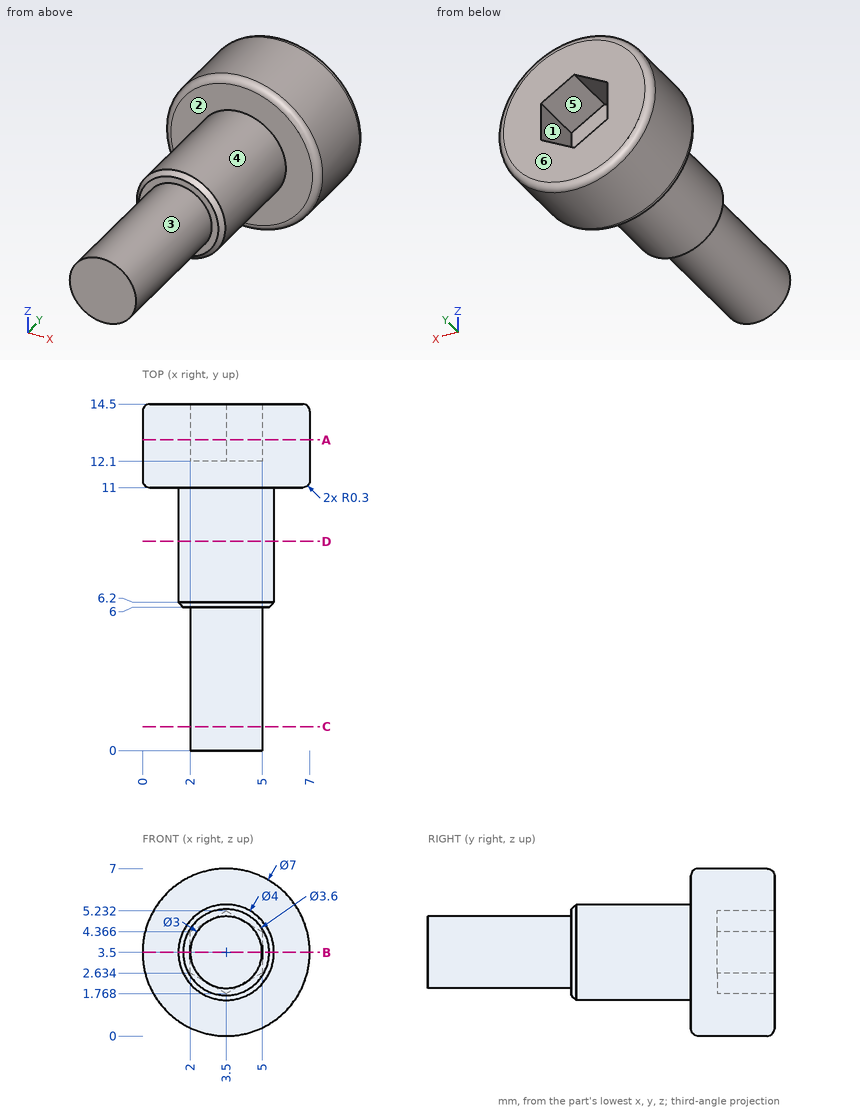
For this review, use the dimensioned drawing (mm, ordinates from the lowest corner) and the shaded views. A direction names the side the tool comes from. Give positions to 0.01 mm unless a question says otherwise; leave off trailing zeros. Order: outer loops, then holes, each group sorted by start corner. A loop starts at its lowest first (then second) coordinate and runs counter-clockwise, first axis right, second up. Notation, with made-up numbers: (51.25, 86.5) - (83.25, 86.5) arc R16 cw to (83.25, 106.5) - close; hole circle Ø6 at (38, -33.5). An arc over 180 degrees is marked (long way). Use a Markdown table: item, result. Add a question column.
(1) Wall thickness on probe 1 along Y at (x, z) = (1.25, 2.25); probe 2 along Y at (x, z) = (3, 3.5); probe 3 along Z at (x, y) = (3, 13.75): over which ranges is each line inside the solid? List them lowest first. Write a range as [from, to].
(2) Add section B-B on z = 3.5. Give the boundary of the cut face in (x, y), then the cut area to 3 significant figures.
(3) Mouldability with a two-part tool opening along Z and no side actions: class the marked faces 1, 2 and 3 as +Z half, -Z half, draft (parallel to the pull), parting line (faces both ways), or undercut.
(4) Add section D-D on y = 8.75. Give the boundary of the cut face in (x, z).
(5) Add section A-A on y = 13. Give the boundary of the cut face in (x, z), then the cut area to 3 significant figures.
(6) Machinability: for the marked faces 4, 5 and 6, which of the approach directions +Z, -Z, +X, -X, +Y, -Y give a long, thin tool a straight path to every point of the face, cutting with its end or side? Answer none if there is none.
(7) Add section C-C on y = 1. Give the boundary of the cut face in (x, z), then the cut area to 3 significant figures.
(8) Clearance check with flat-ended pins moving along their axes: P1, Ø1.5, axis at x = 4, z = 3.5, coming from the +Y side; P2, Ø1.5, axis at y = 4, z = 3.5, coming from the -X side; P3, Ø1, axis at x = 6, z = 4, coming from the -Y side. State where each tip first meets the part, or that it passes through.
Report:
| question | item | result |
|---|---|---|
| 1 | probe 1 | y = [11, 14.5] |
| 1 | probe 2 | y = [0, 12.1] |
| 1 | probe 3 | z = [0.04, 2.06], [4.94, 6.96] |
| 2 | outline | (0, 11.3) arc R0.3 ccw to (0.3, 11) - (1.5, 11) - (1.5, 6.2) - (1.7, 6) - (2, 6) - (2, 0) - (5, 0) - (5, 6) - (5.3, 6) - (5.5, 6.2) - (5.5, 11) - (6.7, 11) arc R0.3 ccw to (7, 11.3) - (7, 14.2) arc R0.3 ccw to (6.7, 14.5) - (5, 14.5) - (5, 12.1) - (2, 12.1) - (2, 14.5) - (0.3, 14.5) arc R0.3 ccw to (0, 14.2) - close |
| 2 | area | 55.2 mm² |
| 3 | face 1 | undercut |
| 3 | face 2 | draft |
| 3 | face 3 | parting line |
| 4 | outline | circle Ø4 at (3.5, 3.5) |
| 5 | outline | circle Ø7 at (3.5, 3.5); hole (2, 2.63) - (3.5, 1.77) - (5, 2.63) - (5, 4.37) - (3.5, 5.23) - (2, 4.37) - close |
| 5 | area | 30.7 mm² |
| 6 | face 4 | -Y |
| 6 | face 5 | +Y |
| 6 | face 6 | +Z, -Z, +X, -X, +Y |
| 7 | outline | circle Ø3 at (3.5, 3.5) |
| 7 | area | 7.07 mm² |
| 8 | P1 | stops at y = 12.1 |
| 8 | P2 | stops at x = 2 |
| 8 | P3 | stops at y = 11 |
